from build123d import *

# Parameters (mm, degrees)
F0_W     = 31.75
F0_H     = 23.876
F0_W_2   = 6.096
F0_H_2   = 1.5875
F1_DEPTH = 22.352
F2_DEPTH = 6.35
F3_D     = 4.318
F5_D     = 3.571875
F6_D     = 3.5814
F6_DEPTH = 4.572
F6_TIP   = 1.0759611105


with BuildPart() as f1:
    # F0 (on Front) → F1 (new body)
    with BuildSketch(Plane.XZ):
        with Locations((15.875, 11.938)):
            Rectangle(F0_W, F0_H)
        with Locations((8.780638318, 18.31975)):
            Rectangle(F0_W_2, F0_H_2, mode=Mode.SUBTRACT)
        with Locations((22.969361682, 18.31975)):
            Rectangle(F0_W_2, F0_H_2, mode=Mode.SUBTRACT)
        with Locations((8.780638318, 18.31975)):
            Rectangle(F0_W_2, F0_H_2)
        with Locations((22.969361682, 18.31975)):
            Rectangle(F0_W_2, F0_H_2)
    extrude(amount=F1_DEPTH)

    # F0 (on Front) → F2 (join)
    with BuildSketch(Plane.XZ):
        with Locations((22.969361682, 18.31975)):
            Rectangle(F0_W_2, F0_H_2)
        with Locations((8.780638318, 18.31975)):
            Rectangle(F0_W_2, F0_H_2)
    extrude(amount=-F2_DEPTH)

    # F3 (through all)
    with Locations(Plane(origin=(0, 0, 0), x_dir=(1, 0, 0), z_dir=(0, 1, 0))):
        with Locations((7.874, -7.874), (23.876, -7.874)):
            Hole(F3_D / 2)

    # F5 (through all)
    with Locations(Plane.XY.offset(23.876)):
        with Locations((15.875, -3.302), (15.875, -19.05)):
            Hole(F5_D / 2)

    # F6
    with Locations(Plane.XY.offset(23.876)):
        with Locations((15.875, -11.176)):
            Hole(F6_D / 2, depth=F6_DEPTH)
            with Locations((0, 0, -(F6_DEPTH + F6_TIP / 2))):  # 118° drill point
                Cone(0, F6_D / 2, F6_TIP, mode=Mode.SUBTRACT)


solid = f1.part
Verification items for the finished model (mm, model axes). A direction names the side the tool comes from. Give positions to 0.01 mm unless a question says otherwise; leave off trailing zeros. Loops run counter-clockwise (first coordinate to the right, second up) from the corner with the lowest first, then second, coordinate; pieces in that order, holes last. Notation, with made-up numbers: (13, 83) - (45, 83) arc R21 ccw to (45, 109) - close; hole circle Ø1 at (6.25, -4). An arc over 180 degrees is marked (long way). Write item = value, one per line. Start each with the question number.
Q1. Cross-section at C-C, the plane y = -19.05. Enter the section's corners in (x, z) (3 decimals).
Q2. Cross-section at D-D, the plane z = 21.25. Enter the section's corners in (x, y) (3 decimals).
Q3. Thickness scan on line 1 (Z direction, x = 24, y = -17.5); line 2 (X direction, y = -7.75, z = 6.5); line 3 (Y direction, x = 24.5, z = 15.75). Record the ranges inside material, lowest first.
Q4. Cross-section at B-B, the plane x = 22.5. Enter the section's corners in (y, z).
Q5. Tool access check on faces 1 (the face through (16.1, -9.4, 21.6)), 2 (the face through (26.017, 3, 18)), 3 (the face through (5.733, 3, 18)). Record the directions out of +Z, -Z, +X, -X, +Y, -Y that give a thin tool (end or side, any length) a straight path to the whole face; none if there is none.
Q6. Depth check by flat-ended pin: P1, Ø4, axis at x = 7.874, z = 7.874, coming from the +Y side; P2, Ø3, axis at x = 9, y = 3, coming from the -Z side; P3, Ø5, axis at x = 27, z = 6, coming from the +Y side; P4, Ø1.7, axis at y = 3, z = 18, coming from the +X side. Enter the tip coordinate at first touch or a pass-through.
Q7. Mould release check, pull along Z, two halves, no side actions. Record for faces 4 (the face through (6.713, -11.332, 6.054)), 5 (the face through (9, 3, 17.526)), 6 (the face through (23, 6.35, 18)), 7 (the face through (23, 3, 19.114)): released by +Z, released by -Z, zero draft, split by the parting line, or undercut.
Q8. Cross-section at A-A, the plane y = 2. Enter the section's corners in (x, z), and give its area (3 significant figures).
Answer key:
q1.outline = (0, 0) - (14.089, 0) - (14.089, 23.876) - (0, 23.876) - close; (17.661, 0) - (31.75, 0) - (31.75, 23.876) - (17.661, 23.876) - close; hole circle Ø4.318 at (7.874, 7.874); hole circle Ø4.318 at (23.876, 7.874)
q2.outline = (0, -22.352) - (31.75, -22.352) - (31.75, 0) - (0, 0) - close; hole circle Ø3.581 at (15.875, -11.176); hole circle Ø3.572 at (15.875, -19.05); hole circle Ø3.572 at (15.875, -3.302)
q3.line_1 = 0 to 5.72, 10.03 to 23.88
q3.line_2 = 0 to 6.21, 9.54 to 22.21, 25.54 to 31.75
q3.line_3 = -22.35 to 0
q4.outline = (-22.35, 0) - (0, 0) - (0, 6.21) - (-22.35, 6.21) - close; (-22.35, 9.54) - (0, 9.54) - (0, 17.53) - (6.35, 17.53) - (6.35, 19.11) - (0, 19.11) - (0, 23.88) - (-22.35, 23.88) - close
q5.face_1 = +Z
q5.face_2 = +Z, -Z, +X, +Y
q5.face_3 = +Z, -Z, -X, +Y
q6.P1 = through
q6.P2 = 17.53
q6.P3 = 0
q6.P4 = 26.02
q7.face_4 = undercut
q7.face_5 = released by -Z
q7.face_6 = zero draft
q7.face_7 = released by +Z
q8.outline = (5.73, 17.53) - (11.83, 17.53) - (11.83, 19.11) - (5.73, 19.11) - close; (19.92, 17.53) - (26.02, 17.53) - (26.02, 19.11) - (19.92, 19.11) - close
q8.area = 19.4 mm^2
